Build history of the part. All positions in model axes, mm. Give positions to 0.01 mm unless a question says otherwise; leave off trailing zeros. Order: outer loops, then holes, each group sorted by start corner. A loop starts at its lowest first (then second) coordinate and runs counter-clockwise, first axis right, second up. Notation, with made-up numbers: (82, 27.5) -> (135, 27.5) arc R13 ccw to (135, 50.5) -> close; hole circle Ø5 at (67, -7). An arc over 180 degrees is marked (long way). One line per question, with ' | ' between items. Start each with the question number.
(1) Pull direction Z, two halves, no side cores. Call faces 1 (the face through (38.787, 2.465, 24.729)), 2 (the face through (1, 5, 20)), 3 (the face through (0.088, 2.465, 43.498)): +Z half, -Z half, draft (parallel to the pull), parting line (faces both ways), or undercut.
(2) Cut at A-A (x = 0). Give the cut face in (y, z), then the cut area to 3 significant figures.
(3) Cut at B-B (y = 0.85). Give the number of separate pieces and of enclosed holes in the cut face, then the cut area to 3 significant figures.
(4) Cut at C-C (x = -23.55). Give the cut face in (y, z), then the cut area to 3 significant figures.
(5) Drill centre lines: L1, parallel to Z at x = -23.55, y = 1.35; L2, parallel to X at y = 1.35, z = 0. Where is each one in solid material? Low to high. Write a range as from..to.
(6) Pin check, flat tips, straight feed: pin 1 Ø6.5 at (x, z) = (23.55, 23.55) entering from +Y; pin 2 Ø2 at (x, z) = (26, 27.5) entering from +Y; pin 3 Ø3 at (x, y) = (26.5, 4.5) entering from -Z. Stop position of each tip, or through.
(7) Cut at D-D (z = 41.5). Give the cut face in (x, y), then the cut area to 3 significant figures.
from build123d import *

# Parameters (mm, degrees)
SKETCH1_R                                    = 46
SKETCH1_R_2                                  = 19.25
SKETCH1_R_3                                  = 2.5
BOSS_EXTRUDE1_DEPTH                          = 5
SKETCH3_R                                    = 2
CUT_EXTRUDE2_DEPTH                           = 66.245689513
SKETCH7_R                                    = 19.5
CUT_EXTRUDE3_DEPTH                           = 66.245689513
CSK_FOR_M5_SOCKET_COUNTERSUNK_HEAD_S_2_COUNT = 2
CSK_FOR_M5_SOCKET_COUNTERSUNK_HEAD_S_2_PITCH = 47.1
CSK_FOR_M5_SOCKET_COUNTERSUNK_HEAD_S_3_COUNT = 2
CSK_FOR_M5_SOCKET_COUNTERSUNK_HEAD_S_3_PITCH = 66.609458788
CSK_FOR_M5_SOCKET_COUNTERSUNK_HEAD_S_4_COUNT = 2
CSK_FOR_M5_SOCKET_COUNTERSUNK_HEAD_S_4_PITCH = 47.1


with BuildPart() as part:
    # Sketch1 → Boss-Extrude1 (new body)
    # profile 1 of 2: a face of its own
    with BuildSketch(Plane(origin=(0, 0, 0), x_dir=(1, 0, 0), z_dir=(0, 1, 0))):
        with Locations(Location((0, 0, 0), (0, 0, 270))):
            Circle(SKETCH1_R)
        Circle(SKETCH1_R_2, mode=Mode.SUBTRACT)
        with Locations(Location((-23.55, -23.55, 0), (0, 0, 270))):
            Circle(SKETCH1_R_3, mode=Mode.SUBTRACT)
        with Locations(Location((23.55, -23.55, 0), (0, 0, 270))):
            Circle(SKETCH1_R_3, mode=Mode.SUBTRACT)
        with Locations(Location((23.55, 23.55, 0), (0, 0, 270))):
            Circle(SKETCH1_R_3, mode=Mode.SUBTRACT)
        with Locations(Location((-23.55, 23.55, 0), (0, 0, 270))):
            Circle(SKETCH1_R_3, mode=Mode.SUBTRACT)
    # profile 2 of 2: a face of its own
    with BuildSketch(Plane(origin=(0, 0, 0), x_dir=(1, 0, 0), z_dir=(0, 1, 0))):
        Circle(SKETCH1_R_2)
    extrude(amount=BOSS_EXTRUDE1_DEPTH)

    # Sketch3 → Cut-Extrude2 (cut, through all)
    with BuildSketch(Plane.XZ):
        with Locations(Location((0, 41.5, 0), (0, 0, 270))):
            Circle(SKETCH3_R)
        with Locations(Location((35.940054257, 20.75, 0), (0, 0, 270))):
            Circle(SKETCH3_R)
        with Locations(Location((35.940054257, -20.75, 0), (0, 0, 270))):
            Circle(SKETCH3_R)
        with Locations(Location((0, -41.5, 0), (0, 0, 270))):
            Circle(SKETCH3_R)
        with Locations(Location((-35.940054257, -20.75, 0), (0, 0, 270))):
            Circle(SKETCH3_R)
        with Locations(Location((-35.940054257, 20.75, 0), (0, 0, 270))):
            Circle(SKETCH3_R)
    extrude(amount=-CUT_EXTRUDE2_DEPTH, mode=Mode.SUBTRACT)

    # Sketch7 → Cut-Extrude3 (cut, through all)
    with BuildSketch(Plane.XZ):
        with Locations(Location((0, 0, 0), (0, 0, 270))):
            Circle(SKETCH7_R)
    extrude(amount=-CUT_EXTRUDE3_DEPTH, mode=Mode.SUBTRACT)

    # Sketch8 → CSK for M5 socket countersunk head screw (revolve, cut)
    with BuildSketch(Plane(origin=(23.55, 5, -23.55), x_dir=(0, 0, 1), z_dir=(1, 0, 0))):
        Polygon((0, 0), (0, 5), (2.75, 5), (2.75, 3.25), (6, 0), align=None)
    csk_for_m5_socket_countersunk_head_screw = revolve(axis=Axis((23.55, 11.35, -23.55), (0, -1, 0)), mode=Mode.SUBTRACT)

    # CSK for M5 socket countersunk head s 2: CSK for M5 socket countersunk head screw ×2
    with Locations(*[(0, 0, i * CSK_FOR_M5_SOCKET_COUNTERSUNK_HEAD_S_2_PITCH) for i in range(1, CSK_FOR_M5_SOCKET_COUNTERSUNK_HEAD_S_2_COUNT)]):
        add(csk_for_m5_socket_countersunk_head_screw, mode=Mode.SUBTRACT)

    # CSK for M5 socket countersunk head s 3: CSK for M5 socket countersunk head screw ×2
    with Locations(*[Vector(-0.7071067811865476, 0, 0.7071067811865476) * (i * CSK_FOR_M5_SOCKET_COUNTERSUNK_HEAD_S_3_PITCH) for i in range(1, CSK_FOR_M5_SOCKET_COUNTERSUNK_HEAD_S_3_COUNT)]):
        add(csk_for_m5_socket_countersunk_head_screw, mode=Mode.SUBTRACT)

    # CSK for M5 socket countersunk head s 4: CSK for M5 socket countersunk head screw ×2
    with Locations(*[(-i * CSK_FOR_M5_SOCKET_COUNTERSUNK_HEAD_S_4_PITCH, 0, 0) for i in range(1, CSK_FOR_M5_SOCKET_COUNTERSUNK_HEAD_S_4_COUNT)]):
        add(csk_for_m5_socket_countersunk_head_screw, mode=Mode.SUBTRACT)


solid = part.part
Result set:
1) face 1: parting line | face 2: draft | face 3: undercut
2) outline: (0, -46) -> (5, -46) -> (5, -43.5) -> (0, -43.5) -> close; (0, -39.5) -> (5, -39.5) -> (5, -19.5) -> (0, -19.5) -> close; (0, 19.5) -> (5, 19.5) -> (5, 39.5) -> (0, 39.5) -> close; (0, 43.5) -> (5, 43.5) -> (5, 46) -> (0, 46) -> close | area: 225 mm2
3) separate pieces: 1 | enclosed holes: 11 | area: 5,280 mm2
4) outline: (0, -39.51) -> (5, -39.51) -> (5, -29.55) -> (1.75, -26.3) -> (0, -26.3) -> close; (0, -20.8) -> (1.75, -20.8) -> (5, -17.55) -> (5, 17.55) -> (1.75, 20.8) -> (0, 20.8) -> close; (0, 26.3) -> (1.75, 26.3) -> (5, 29.55) -> (5, 39.51) -> (0, 39.51) -> close | area: 319 mm2
5) L1: z = -39.51..-26.3, -20.8..20.8, 26.3..39.51 | L2: x = -46..-19.5, 19.5..46
6) pin 1: stops at y = 2.25 | pin 2: stops at y = 4.65 | pin 3: stops at z = -38.61
7) outline: (-19.84, 0) -> (-2, 0) -> (-2, 5) -> (-19.84, 5) -> close; (2, 0) -> (19.84, 0) -> (19.84, 5) -> (2, 5) -> close | area: 178 mm2
